Autodesk Inventor part; units mm, degrees
ref_plane "YZ Plane" through (0, 0, 0) normal (1, 0, 0) x (0, 1, 0)
ref_plane "XZ Plane" through (0, 0, 0) normal (0, 1, 0) x (-1, 0, 0)
ref_plane "XY Plane" through (0, 0, 0) normal (0, 0, 1) x (1, 0, 0)
sketch "Sketch1" plane through (0, 0, 0) normal (0, 0, 1) x (1, 0, 0)
  circle A0 centre (11.9062, -20.6222) radius 2.5908 construction
  circle A1 centre (-23.8125, 0) radius 2.5908 construction
  circle A2 centre (11.9063, 20.6222) radius 2.5908
  circle A3 centre (23.8125, 0) radius 2.5908 construction
  circle A4 centre (-11.9062, 20.6222) radius 2.5908
  circle A5 centre (-11.9062, -20.6222) radius 2.5908 construction
  circle A6 centre (0, 0) radius 14.478 construction
  circle A7 centre (57.15, 98.9867) radius 3.175
  circle A8 centre (69.85, 120.9837) radius 3.175
  circle A9 centre (98.9867, 57.15) radius 3.175 construction
  circle A10 centre (120.9837, 69.85) radius 3.175 construction
  circle A11 centre (114.3, 0) radius 3.175 construction
  circle A12 centre (139.7, 0) radius 3.175 construction
  circle A13 centre (98.9867, -57.15) radius 3.175 construction
  circle A14 centre (120.9837, -69.85) radius 3.175 construction
  circle A15 centre (57.15, -98.9867) radius 3.175 construction
  circle A16 centre (69.85, -120.9837) radius 3.175 construction
  circle A17 centre (0, -114.3) radius 3.175 construction
  circle A18 centre (0, -139.7) radius 3.175 construction
  circle A19 centre (-57.15, -98.9867) radius 3.175 construction
  circle A20 centre (-69.85, -120.9837) radius 3.175 construction
  circle A21 centre (-98.9867, -57.15) radius 3.175 construction
  circle A22 centre (-120.9837, -69.85) radius 3.175 construction
  circle A23 centre (-114.3, 0) radius 3.175 construction
  circle A24 centre (-139.7, 0) radius 3.175 construction
  circle A25 centre (-98.9867, 57.15) radius 3.175 construction
  circle A26 centre (-120.9837, 69.85) radius 3.175 construction
  circle A27 centre (-57.15, 98.9867) radius 3.175 construction
  circle A28 centre (-69.85, 120.9837) radius 3.175 construction
  circle A29 centre (0, 114.3) radius 3.175 construction
  circle A30 centre (0, 139.7) radius 3.175 construction
  circle A31 centre (0, 0) radius 152.4 construction
  arc A32 (92.1001, 121.4221) -> (59.1046, 140.4721) centre (0, 0) ccw
  line L0 (59.1046, 140.4721) -> (0, 38.1)
  line L1 (92.1001, 121.4221) -> (32.9956, 19.05)
  line L2 (69.85, 120.9837) -> (0, 0) construction
  line L3 (0, 0) -> (-12.5383, 7.239) construction
  line L4 (0, -263.7526) -> (0, 221.7588) construction
  arc A33 (0, 38.1) -> (-32.9956, 19.05) centre (0, 0) ccw
  line L5 (12.5383, 7.239) -> (0, 0) construction
  arc A34 (13.9131, 8.0328) -> (-13.9131, 8.0328) centre (0, 0) ccw
  line L6 (-13.9131, 8.0328) -> (-32.9956, 19.05)
  line L7 (32.9956, 19.05) -> (13.9131, 8.0328)
  dimension "d1" = 38.1
  dimension "d19" = 1.5875
extrude "Extrusion1" add sketch "Sketch1" along normal blind 6.35
sketch "Sketch2" plane through (0, 0, 6.35) normal (0, 0, 1) x (1, 0, 0)
  line L0 (12.0202, 46.2196) -> (26.5051, 71.3083)
  line L1 (32.4298, 69.7208) -> (32.4298, 36.2693)
  line L2 (27.6673, 33.5196) -> (13.1824, 41.8825)
  line L3 (59.1046, 140.4721) -> (0, 38.1) construction
  arc A0 (0, 38.1) -> (-32.9956, 19.05) centre (0, 0) ccw construction
  line L4 (38.7798, 87.0693) -> (38.7798, 53.6178)
  line L5 (43.5423, 89.8189) -> (58.0272, 81.456)
  line L6 (59.1893, 77.1189) -> (44.7044, 52.0303)
  line L7 (32.9956, 19.05) -> (92.1001, 121.4221) construction
  circle A1 centre (11.9063, 20.6222) radius 2.5908 construction
  arc A2 (12.0202, 46.2196) -> (13.1824, 41.8825) centre (14.7699, 44.6321) ccw
  arc A3 (32.4298, 69.7208) -> (26.5051, 71.3083) centre (29.2548, 69.7208) ccw
  arc A4 (27.6673, 33.5196) -> (32.4298, 36.2693) centre (29.2548, 36.2693) ccw
  arc A5 (38.7798, 53.6178) -> (44.7044, 52.0303) centre (41.9548, 53.6178) ccw
  arc A6 (43.5423, 89.8189) -> (38.7798, 87.0693) centre (41.9548, 87.0693) ccw
  arc A7 (59.1893, 77.1189) -> (58.0272, 81.456) centre (56.4397, 78.7064) ccw
  point P0 (0, 0)
  point P1 (32.4298, 30.77)
  point P2 (38.7798, 92.5685)
  dimension "d4" = 6.35
  dimension "d5" = 6.35
  dimension "d6" = 6.35
  dimension "d7" = 19.05
  dimension "d8" = 3.175
extrude "Extrusion2" cut sketch "Sketch2" against normal blind 6.35
sketch "Sketch3" plane through (0, 0, 6.35) normal (0, 0, 1) x (1, 0, 0)
  circle A0 centre (32.4298, 81.57) radius 3.175
  line L0 (12.0202, 46.2196) -> (26.5051, 71.3083) construction
  circle A1 centre (38.7798, 41.7685) radius 3.175
  line L1 (59.1893, 77.1189) -> (44.7044, 52.0303) construction
  line L2 (32.4298, 69.7208) -> (32.4298, 36.2693) construction
  line L3 (38.7798, 53.6178) -> (38.7798, 87.0693) construction
  point P0 (0, 0)
  dimension "d12" = 6.35
extrude "Extrusion3" cut sketch "Sketch3" against normal through all
sketch "Sketch4" plane through (0, 0, 6.35) normal (0, 0, 1) x (1, 0, 0)
  arc A0 (32.4298, 94.27) -> (21.4313, 75.22) centre (32.4298, 81.57) ccw
  circle A1 centre (32.4298, 81.57) radius 3.175 construction
  line L0 (32.4298, 94.27) -> (21.4313, 75.22)
  line L1 (59.1046, 140.4721) -> (0, 38.1) construction
  arc A2 (38.7798, 29.0685) -> (49.7783, 48.1185) centre (38.7798, 41.7685) ccw
  line L2 (49.7783, 48.1185) -> (38.7798, 29.0685)
  circle A3 centre (38.7798, 41.7685) radius 3.175 construction
  line L3 (32.9956, 19.05) -> (92.1001, 121.4221) construction
  point P0 (0, 0)
  point P1 (57.6913, 138.0243)
  point P2 (0.8924, 39.6457)
  point P3 (33.4209, 19.7868)
  point P4 (90.6869, 118.9743)
  dimension "d15" = 12.7
extrude "Extrusion4" add sketch "Sketch4" against normal blind 6.35
fillet "Fillet2" radius 3.175 11 edges at (-32.9956, 19.05, 3.175) (0, 38.1, 3.175) (32.4298, 94.27, 3.175) (21.4313, 75.22, 3.175) (59.1046, 140.4721, 3.175) (92.1001, 121.4221, 3.175) (49.7783, 48.1185, 3.175) (38.7798, 29.0685, 3.175) (32.9956, 19.05, 3.175) (-13.9131, 8.0328, 3.175) (13.9131, 8.0328, 3.175)
equation "\"d5\" = d4"
equation "\"d6\" = d4"
properties part number "Doubler" material "Aluminum 6061"
Part model, mm, in its own coordinate system. A direction names the side the tool comes from. Coordinates: 2 decimals unless noted, no trailing zeros. Order: outer loops, then holes, each group sorted by start corner. A loop starts at its lowest first (then second) coordinate and runs counter-clockwise, first axis right, second up. Notation, with made-up numbers: M 12,58 L 24,58 A14 ccw 24,70 Z; hole C -20,42.25 d4. An arc over 180 degrees is marked long. One line per question, with ' | ' between items.
Q1. 3-axis set-ups, long thin cutter, end or side, ignore diameter. For faces 5 (the face through (11.694, 43.844, 3.219)), 6 (the face through (49.695, 35.276, 3.219)): which of +Z, -Z, +X, -X, +Y, -Y reach the whole face in a straight line?
A:
face 5: +Z, -Z | face 6: +Z, -Z, +X
Q2. Drill centre lines: line 1 (X direction, y = 81.5, z = 0.75); line 2 (X direction, y = 40, z = 4); line 3 (Y direction, x = 57.15, z = 1.75). Where is each one in solid material? Low to high.
A:
line 1: x = 19.73 to 29.26, 35.6 to 38.78, 57.95 to 69.05 | line 2: x = 1.1 to 16.44, 32.43 to 36.14, 41.42 to 51.36 | line 3: y = 60.89 to 73.59, 81.96 to 95.81, 102.16 to 137.09
Q3. Slice it at C-C (z = 2.5). Count the separate pieces of the cut face and the enclosed holes in it, and give its area (3 significant figures).
A:
separate pieces: 1 | enclosed holes: 8 | area: 4,620 mm^2
Q4. Two-plate mould, pull along X, no slides. Class faces 1 (the face through (41.077, 50.567, 3.219)), 2 (the face through (-23.182, 13.384, 3.131)), 3 (the face through (91.05, 121.19, 3.22)), 4 (the face through (59.515, 79.494, 3.219)): +X half, -X half, draft (parallel to the pull), parting line (faces both ways), or undercut.
A:
face 1: undercut | face 2: -X half | face 3: +X half | face 4: undercut
Q5. Slice it at A-A (y = 64). Give the cut face in (x, z).
A:
outline: M 14.95,0 L 22.29,0 L 22.29,6.35 L 14.95,6.35 Z; M 32.43,0 L 38.78,0 L 38.78,6.35 L 32.43,6.35 Z; M 51.62,0 L 58.95,0 L 58.95,6.35 L 51.62,6.35 Z
Q6. Slice it at D-D (x = 82.5). Give the cut face in (y, z), and give its area (3 significant figures).
A:
outline: M 104.79,0 L 128.14,0 L 128.14,6.35 L 104.79,6.35 Z | area: 148 mm^2
Q7. Pin check, flat tips, straight feed: P1, Ø1.9, axis at y = 45, z = 3, coming from the -X side; P2, Ø1.5, axis at x = 66, z = 2, coming from the -Y side; P3, Ø2, axis at x = 61.5, z = 2.5, coming from the -Y side. Stop position of each tip, or through.
A:
P1: stops at x = 3.44 | P2: stops at y = 74.92 | P3: stops at y = 66.69
Q8. Slice it at B-B (x = 69.85). Give the cut face in (y, z).
A:
outline: M 82.88,0 L 117.81,0 L 117.81,6.35 L 82.88,6.35 Z; M 124.16,0 L 135.45,0 L 135.45,6.35 L 124.16,6.35 Z
